```python
from build123d import *

# Parameters (mm, degrees)
BASE_FLANGE1_DEPTH        = 5.08
TAIL_CONNECTION_DEPTH     = 2.54
SKETCH4_R                 = 4.064
TAB_BOLT_HOLES_DEPTH      = 184.232438176
BATTERY_CUTOUT_DEPTH      = 2.54
SKETCH6_W                 = 6.35
SKETCH6_H                 = 49.280438222
TOP_WIRE_CONNECTION_DEPTH = 2.54
SKETCH7_W                 = 6.35
SKETCH7_H                 = 6.091561778
BOTTOM_WIRES_DEPTH        = 2.54
SKETCH8_R                 = 2.286
BOTTOM_BOLTS_DEPTH        = 184.232438176
CUT_EXTRUDE10_DEPTH       = 1.5875


# Sheet-metal steps are written as plain solids
with BuildPart() as part:
    # Sketch1 → Base-Flange1 (new body)
    with BuildSketch(Plane.XY):
        Polygon((0, 0), (46.99, 0), (101.6, 72.644), (101.6, 152.4), (-101.6, 152.4), (-101.6, 72.644), (-46.99, 0), align=None)
    extrude(amount=-BASE_FLANGE1_DEPTH)

    # Sketch2 → Tail Connection (cut)
    with BuildSketch(Plane.XY):
        with BuildLine():
            Line((-5.969, 137.668), (5.969, 137.668))
            ThreePointArc((5.969, 137.668), (13.462, 130.175), (5.969, 122.682))
            Line((5.969, 122.682), (-5.969, 122.682))
            ThreePointArc((-5.969, 122.682), (-13.462, 130.175), (-5.969, 137.668))
        make_face()
    extrude(amount=-TAIL_CONNECTION_DEPTH, mode=Mode.SUBTRACT)

    # Sketch4 → Tab Bolt Holes (cut, through all)
    with BuildSketch(Plane.XY):
        with Locations((-85.852, 130.175)):
            Circle(SKETCH4_R)
        with Locations((85.852, 130.175)):
            Circle(SKETCH4_R)
    extrude(amount=-TAB_BOLT_HOLES_DEPTH, mode=Mode.SUBTRACT)

    # Sketch5 → Battery Cutout (cut)
    with BuildSketch(Plane.XY):
        Polygon((-76.973649394, 50.672541858), (-76.973649394, 73.401561778), (77.43879929, 73.401561778), (77.43879929, 49.679437927), (45.952574948, 6.091561778), (-45.487425052, 6.091561778), align=None)
    extrude(amount=-BATTERY_CUTOUT_DEPTH, mode=Mode.SUBTRACT)

    # Sketch6 → Top Wire Connection (cut)
    with BuildSketch(Plane.XY):
        with Locations((0, 98.041780889)):
            Rectangle(SKETCH6_W, SKETCH6_H)
    extrude(amount=-TOP_WIRE_CONNECTION_DEPTH, mode=Mode.SUBTRACT)

    # Sketch7 → Bottom Wires (cut)
    with BuildSketch(Plane.XY):
        with Locations((0, 3.045780889)):
            Rectangle(SKETCH7_W, SKETCH7_H)
    extrude(amount=-BOTTOM_WIRES_DEPTH, mode=Mode.SUBTRACT)

    # Sketch8 → Bottom Bolts (cut, through all)
    with BuildSketch(Plane.XY):
        with Locations((-82.053649394, 67.056)):
            Circle(SKETCH8_R)
        with Locations((82.51879929, 67.056)):
            Circle(SKETCH8_R)
    extrude(amount=-BOTTOM_BOLTS_DEPTH, mode=Mode.SUBTRACT)

    # Sketch9 → Cut-Extrude10 (cut)
    with BuildSketch(Plane.XY):
        with BuildLine():
            Line((72.3265, 152.4), (72.3265, 130.175))
            ThreePointArc((72.3265, 130.175), (85.852, 116.6495), (99.3775, 130.175))
            Line((99.3775, 130.175), (99.3775, 152.4))
            Line((99.3775, 152.4), (72.3265, 152.4))
        make_face()
    cut_extrude10 = extrude(amount=-CUT_EXTRUDE10_DEPTH, mode=Mode.SUBTRACT)

    # Mirror1: Cut-Extrude10 across plane
    add(cut_extrude10.mirror(Plane(origin=(0, 0, 0), x_dir=(0, 0, 1), z_dir=(1, 0, 0))), mode=Mode.SUBTRACT)


solid = part.part
```
Geometry check sheet. Reference: the model listing, model coordinates, mm. A direction names the side the tool comes from. Round coordinates to 2 decimals unless told otherwise and drop trailing zeros. Order: outer loops, then holes, each group sorted by start corner. A loop starts at its lowest first (then second) coordinate and runs counter-clockwise, first axis right, second up. Notation, with made-up numbers: (-1.5, 40) - (53.5, 40) arc R17 ccw to (53.5, 67) - close; hole circle Ø6 at (40, 66.5). An arc over 180 degrees is marked (long way). Use a Markdown table: item, result. Add a question column.
1) Gauge pin test, flat ends, axial feed: P1, Ø6.5, axis at x = -85.852, y = 130.175, coming from the -Z side; P2, Ø3, axis at y = 2, z = -0.5, coming from the +X side; P3, Ø8, axis at x = 79, y = 141, coming from the +Z side; P4, Ø0.8, axis at y = 4, z = -1, coming from the -X side. Record the tip position at first contact, or that the pin passes through.
2) Section check A-A (y = 97.5). Record the cut outline in (x, z) (3 decimals).
3) Section check B-B (x = -40). Record the cut outline in (y, z).
4) Thickness scan on line 1 along X through (y, z) = (98, -2.4) (3 decimals); line 2 along X through (y, z) = (65.5, -1.35); line 3 along Y through (x, z) = (26, -0.65). Record the ranges inside material, lowest first.
5) Section check C-C (z = -3.5). Record the cut outline in (x, y) (3 decimals), then the cut area to 3 significant figures.
6) Mould release check, pull along Y, two halves, no side actions. Record for faces 1 (the flat face through (73.91, 35.81, -2.5)), 2 (the flat face through (-101.6, 113, -3)), 3 (the cylindrical face through (13.46, 130.34, -1.25)), 4 (the cylindrical face through (-83.74, 68.6, -2.5)): released by +Y, released by -Y, zero draft, split by the parting line, or undercut.
7) Set-up check for faces 5 (the cylindrical face through (85.555, 116.653, -0.783)), 6 (the cylindrical face through (84.7, 67.74, -2.5)), 7 (the flat face through (61.916, 28.191, -1.252)): record each of +Z, -Z, +X, -X, +Y, -Y from which the full face is reachable in a straight line by a thin tool's end or side.
Established:
| question | item | result |
|---|---|---|
| 1 | P1 | through |
| 1 | P2 | x = 49.62 |
| 1 | P3 | z = -1.59 |
| 1 | P4 | x = -50.3 |
| 2 | outline | (-101.6, -5.08) - (101.6, -5.08) - (101.6, 0) - (3.175, 0) - (3.175, -2.54) - (-3.175, -2.54) - (-3.175, 0) - (-101.6, 0) - close |
| 3 | outline | (0, -5.08) - (152.4, -5.08) - (152.4, 0) - (73.4, 0) - (73.4, -2.54) - (6.09, -2.54) - (6.09, 0) - (0, 0) - close |
| 4 | line 1 | -101.6 to -3.175, 3.175 to 101.6 |
| 4 | line 2 | -96.23 to -83.73, -80.38 to -76.97, 77.44 to 80.84, 84.19 to 96.23 |
| 4 | line 3 | 0 to 6.09, 73.4 to 152.4 |
| 5 | outline | (-101.6, 72.644) - (-46.99, 0) - (46.99, 0) - (101.6, 72.644) - (101.6, 152.4) - (-101.6, 152.4) - close; hole circle Ø8.128 at (-85.852, 130.175); hole circle Ø4.572 at (-82.054, 67.056); hole circle Ø4.572 at (82.519, 67.056); hole circle Ø8.128 at (85.852, 130.175) |
| 5 | area | 26,900 mm2 |
| 6 | face 1 | released by -Y |
| 6 | face 2 | zero draft |
| 6 | face 3 | undercut |
| 6 | face 4 | undercut |
| 7 | face 5 | +Z, +Y |
| 7 | face 6 | +Z, -Z |
| 7 | face 7 | +Z |
